Geometry check sheet. Reference: the model listing, model coordinates, mm. Face numbers are marked on the shaded views. A direction names the side the tool comes from. Give positions to 0.01 mm unless a question says otherwise; leave off trailing zeros. Order: outer loops, then holes, each group sorted by start corner. A loop starts at its lowest first (then second) coordinate and runs counter-clockwise, first axis right, second up.
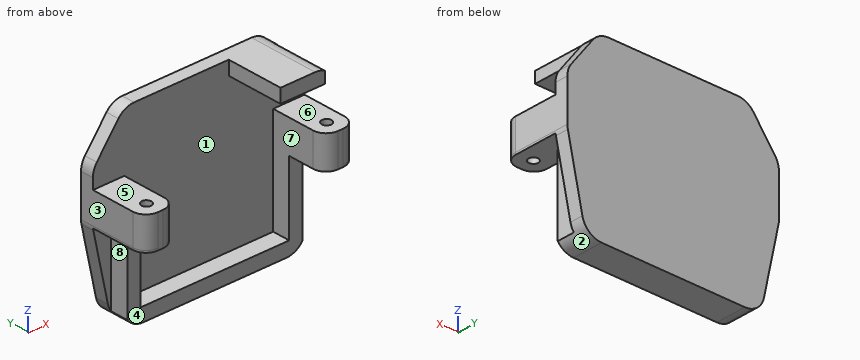
from build123d import *

# Parameters (mm, degrees)
BOSS_EXTRUDE1_START     = -14.7
BOSS_EXTRUDE1_OUTLINE_W = 32.4
BOSS_EXTRUDE1_OUTLINE_H = 27.1
BOSS_EXTRUDE1_DEPTH     = 14.7
CUT_EXTRUDE1_DEPTH      = 12.7
MOVE_FACE1_BY           = 4
MOVE_FACE1_2_BY         = 4
SKETCH3_W               = 2.8
SKETCH3_H               = 13.1
CUT_EXTRUDE2_DEPTH      = 13.7
CUT_EXTRUDE3_DEPTH      = 6
SKETCH5_R               = 0.75
CUT_EXTRUDE4_DEPTH      = 43.343439739
BOSS_EXTRUDE2_DEPTH     = 2
FILLET1_R               = 3
FILLET2_R               = 3
FILLET3_START           = -21
FILLET3_DEPTH           = 13
FILLET4_START           = -21
FILLET4_DEPTH           = 13
FILLET5_R               = 3
FILLET6_R               = 3
FILLET7_R               = 2


with BuildPart() as part:
    # Boss-Extrude1: read off the stored shape, not the designer's step
    # Boss-Extrude1 outline → Boss-Extrude1 (new body)
    with BuildSketch(Plane.XZ.offset(24.012143299).offset(BOSS_EXTRUDE1_START)):
        with Locations((16.432361385, -27.739579566)):
            Rectangle(BOSS_EXTRUDE1_OUTLINE_W, BOSS_EXTRUDE1_OUTLINE_H)
    extrude(amount=BOSS_EXTRUDE1_DEPTH)

    # Sketch2 → Cut-Extrude1 (cut)
    with BuildSketch(Plane.XZ.offset(24.012143299)):
        Polygon((27.832361385, -23.189579566), (32.632361385, -23.189579566), (32.632361385, -20.589579566), (27.832361385, -20.589579566), (27.832361385, -16.289579566), (5.032361385, -16.289579566), (5.032361385, -20.589579566), (0.232361385, -20.589579566), (0.232361385, -23.189579566), (5.032361385, -23.189579566), (5.032361385, -39.189579566), (27.832361385, -39.189579566), align=None)
    extrude(amount=-CUT_EXTRUDE1_DEPTH, mode=Mode.SUBTRACT)

    # Move Face1: a face moved inward by 4.0
    extrude(part.faces().sort_by_distance((16.432361385, -24.012143299, -39.479579566))[0], amount=MOVE_FACE1_BY, dir=(0, 1, 0), mode=Mode.SUBTRACT)

    # Move Face1 2: a face moved inward by 4.0
    extrude(part.faces().sort_by_distance((16.432361385, -24.012143299, -15.789579566))[0], amount=MOVE_FACE1_2_BY, dir=(0, 1, 0), mode=Mode.SUBTRACT)

    # Sketch3 → Cut-Extrude2 (cut)
    with BuildSketch(Plane.XZ.offset(20.012143299)):
        with Locations((1.632361385, -34.739579566)):
            Rectangle(SKETCH3_W, SKETCH3_H)
        with Locations((31.232361385, -34.739579566)):
            Rectangle(SKETCH3_W, SKETCH3_H)
        Polygon((0.232361385, -20.589579566), (5.032361385, -20.589579566), (5.032361385, -16.289579566), (21.032361385, -16.289579566), (21.032361385, -14.189579566), (0.232361385, -14.189579566), align=None)
        Polygon((27.832361385, -14.189579566), (32.632361385, -14.189579566), (32.632361385, -20.589579566), (27.832361385, -20.589579566), (27.832361385, -16.289579566), align=None)
    extrude(amount=-CUT_EXTRUDE2_DEPTH, mode=Mode.SUBTRACT)

    # Sketch4 → Cut-Extrude3 (cut)
    with BuildSketch(Plane.XZ.offset(20.012143299)):
        Polygon((3.032361385, -28.189579566), (5.032361385, -28.189579566), (5.032361385, -39.189579566), (27.832361385, -39.189579566), (27.832361385, -28.189579566), (29.832361385, -28.189579566), (29.832361385, -41.289579566), (3.032361385, -41.289579566), align=None)
    extrude(amount=-CUT_EXTRUDE3_DEPTH, mode=Mode.SUBTRACT)

    # Sketch5 → Cut-Extrude4 (cut, through all)
    with BuildSketch(Plane.XY.offset(-23.189579566)):
        with Locations((2.632361385, -17.662143299)):
            Circle(SKETCH5_R)
        with Locations((30.232361385, -17.662143299)):
            Circle(SKETCH5_R)
    extrude(amount=-CUT_EXTRUDE4_DEPTH, mode=Mode.SUBTRACT)

    # Sketch6 → Boss-Extrude2 (add)
    with BuildSketch(Plane(origin=(0, -9.312143299, 0), x_dir=(1, 0, 0), z_dir=(0, 1, 0))):
        Polygon((21.032361385, 14.189579566), (5.032361385, 14.189579566), (0.232361385, 20.589579566), (5.032361385, 20.589579566), (5.032361385, 16.289579566), (21.032361385, 16.289579566), align=None)
        Polygon((0.232361385, 28.189579566), (3.032361385, 41.289579566), (3.032361385, 28.189579566), align=None)
        Polygon((29.832361385, 41.289579566), (29.832361385, 28.189579566), (32.632361385, 28.189579566), align=None)
        Polygon((27.832361385, 20.589579566), (27.832361385, 14.189579566), (32.632361385, 20.589579566), align=None)
    extrude(amount=-BOSS_EXTRUDE2_DEPTH)

    # Fillet1
    # the kernel refuses this fillet: 3 mm, written as the material it takes off along each edge
    with BuildSketch(Plane(origin=(29.832361385, -17.378495337, -41.289579566), x_dir=(0.20901925718607187, 0, 0.9779115246919747), z_dir=(0, 1, 0))) as fillet1_piece_1:
        with BuildLine():
            CenterArc((FILLET1_R * 0.808846938434, -FILLET1_R), FILLET1_R, 90, 77.935115589)
            Line((-FILLET1_R * 0.169064586258, -FILLET1_R * 0.790980742814), (0, 0))
            Line((0, 0), (FILLET1_R * 0.808846938434, 0))
        make_face()
    extrude(amount=14.132704077, mode=Mode.SUBTRACT)

    # Fillet2
    # the kernel refuses this fillet: 3 mm, written as the material it takes off along each edge
    with BuildSketch(Plane(origin=(3.032361385, -17.378495337, -41.289579566), x_dir=(1.0, 0, -8.828560948914946e-12), z_dir=(0, 1, 0))) as fillet2_piece_1:
        with BuildLine():
            CenterArc((FILLET2_R * 0.808846938434, -FILLET2_R), FILLET2_R, 89.999999999, 77.935115589)
            Line((-FILLET2_R * 0.169064586256, -FILLET2_R * 0.790980742805), (0, 0))
            Line((0, 0), (FILLET2_R * 0.808846938443, 0))
        make_face()
    extrude(amount=14.132704077, mode=Mode.SUBTRACT)

    # Fillet3: read off the stored shape, not the designer's step
    # Fillet3 outline → Fillet3 (cut)
    with BuildSketch(Plane(origin=(0, 0, 0), x_dir=(1, 0, 0), z_dir=(0, 1, 0)).offset(FILLET3_START)):
        with BuildLine():
            Line((0.232361385, 28.189579566), (0.232361385, 27.872549323))
            ThreePointArc((0.232361385, 27.872549323), (0.248973736, 28.187824027), (0.29862681, 28.499607094))
            Line((0.29862681, 28.499607094), (0.232361385, 28.189579566))
        make_face()
    extrude(amount=FILLET3_DEPTH, mode=Mode.SUBTRACT)

    # Fillet4: read off the stored shape, not the designer's step
    # Fillet4 outline → Fillet4 (cut)
    with BuildSketch(Plane(origin=(0, 0, 0), x_dir=(1, 0, 0), z_dir=(0, 1, 0)).offset(FILLET4_START)):
        with BuildLine():
            Line((32.632361385, 28.189579566), (32.566095959, 28.499607094))
            ThreePointArc((32.566095959, 28.499607094), (32.615749033, 28.187824027), (32.632361385, 27.872549323))
            Line((32.632361385, 27.872549323), (32.632361385, 28.189579566))
        make_face()
    extrude(amount=FILLET4_DEPTH, mode=Mode.SUBTRACT)

    # Fillet5
    fillet5_edges = [part.edges().sort_by_distance(p)[0] for p in [
        (32.632361385, -10.312143299, -20.589579566),
        (5.032361385, -10.312143299, -14.189579566),
        (0.232361385, -10.312143299, -20.589579566),
    ]]
    fillet(fillet5_edges, radius=FILLET5_R)

    # Fillet6
    # the kernel refuses this fillet: 3 mm, written as the material it takes off along each edge
    with BuildSketch(Plane(origin=(27.832361385, -20.312143299, -14.189579566), x_dir=(-1.0, 0, -1.4283093226823923e-11), z_dir=(0, 1, 0))) as fillet6_piece_1:
        with BuildLine():
            CenterArc((FILLET6_R * 0.500000000009, -FILLET6_R), FILLET6_R, 90.000000001, 53.130102354)
            Line((-FILLET6_R * 0.3, -FILLET6_R * 0.400000000011), (-FILLET6_R * 0.316, -FILLET6_R * 0.388000000012))
            Line((-FILLET6_R * 0.316, -FILLET6_R * 0.388000000012), (-FILLET6_R * 0.0100000000003, FILLET6_R * 0.0199999999999))
            Line((-FILLET6_R * 0.0100000000003, FILLET6_R * 0.0199999999999), (FILLET6_R * 0.499999999994, FILLET6_R * 0.02))
            Line((FILLET6_R * 0.499999999994, FILLET6_R * 0.02), (FILLET6_R * 0.499999999995, 0))
        make_face()
    extrude(amount=20, mode=Mode.SUBTRACT)

    # Fillet7
    fillet7_edges = [part.edges().sort_by_distance(p)[0] for p in [
        (0.232361385, -20.012143299, -25.531064444),
        (27.832361385, -20.012143299, -25.689579566),
        (0.236563927, -20.012143299, -28.031286811),
        (32.632361385, -20.012143299, -25.531064444),
        (32.628158843, -20.012143299, -28.031286811),
        (5.032361385, -20.012143299, -25.689579566),
    ]]
    fillet(fillet7_edges, radius=FILLET7_R)


solid = part.part
Item 1: Sectioned sample at B-B (z = -27). Enter the section's corners in (x, y).
Reported:
outline: (0.23, -18.01) arc R2 ccw to (2.23, -20.01) - (3.03, -20.01) arc R2 ccw to (5.03, -18.01) - (5.03, -11.31) - (27.83, -11.31) - (27.83, -18.01) arc R2 ccw to (29.83, -20.01) - (30.63, -20.01) arc R2 ccw to (32.63, -18.01) - (32.63, -9.31) - (0.23, -9.31) - close; hole circle Ø1.5 at (2.63, -17.66); hole circle Ø1.5 at (30.23, -17.66)
Item 2: Sectioned sample at C-C (x = 25.5). Enter the section's corners in (y, z), and give its area (3 significant figures).
Reported:
outline: (-20.01, -16.29) - (-11.31, -16.29) - (-11.31, -39.19) - (-14.01, -39.19) - (-14.01, -41.29) - (-9.31, -41.29) - (-9.31, -14.19) - (-20.01, -14.19) - close
area: 78.1 mm2
Item 3: Set-up check for the marked faces 1, 2, 3, 4 and 5: record each of +Z, -Z, +X, -X, +Y, -Y from which the full face is reachable in a straight line by a thin tool's end or side.
Reported:
face 1: -Y
face 2: -Z, +X, +Y, -Y
face 3: +Z, -Z, -X, +Y, -Y
face 4: -Z, +X, -X, -Y
face 5: +Z, +X, -X, -Y
Item 4: Scan lines: L1, parallel to X at y = -11.75, z = -26; L2, parallel to Z at x = 25.5, y = -11.75; L3, parallel to X at y = -12.5, z = -34.75. Record each from-to range of solid material in increasing order.
Reported:
L1: x = 0.23 to 5.03, 27.83 to 32.63
L2: z = -41.29 to -39.19, -16.29 to -14.19
L3: x = 3.03 to 5.03, 27.83 to 29.83
Item 5: Sectioned sample at D-D (y = -10.5). Enter the section's corners in (x, z), and give its area (3 significant figures).
Reported:
outline: (0.23, -27.87) arc R3 ccw to (0.3, -28.5) - (2.53, -38.92) arc R3 ccw to (5.46, -41.29) - (27.41, -41.29) arc R3 ccw to (30.34, -38.92) - (32.57, -28.5) arc R3 ccw to (32.63, -27.87) - (32.63, -21.59) arc R3 ccw to (32.03, -19.79) - (28.73, -15.39) arc R3 ccw to (26.33, -14.19) - (6.53, -14.19) arc R3 ccw to (4.13, -15.39) - (0.83, -19.79) arc R3 ccw to (0.23, -21.59) - close
area: 807 mm2
Item 6: Gauge pin test, flat ends, axial feed: pin 1 (5.5 mm diameter, centred on x = 31, y = -15.5, fed in from -Z); pin 2 (1.4 mm diameter, centred on x = 3.5, y = -15.5, fed in from +Z); pin 3 (6.5 mm diameter, centred on x = 10.5, z = -36.5, fed in from -Y); pin 4 (2 mm diameter, centred on y = -14, z = -20.5, fed in from +X). Record the tip position at first contact, or that the pin passes through.
Reported:
pin 1: stops at z = -41
pin 2: stops at z = -23.19
pin 3: stops at y = -14.01
pin 4: passes through
Item 7: Draft check along X on the marked faces 6, 7 and 8. Enter one of: released by +X, released by -X, zero draft, split by the parting line, or undercut.
Reported:
face 6: zero draft
face 7: undercut
face 8: released by -X
Item 8: Sectioned sample at A-A (y = -14.5). Enter the section's corners in (x, z), and give its area (3 significant figures).
Reported:
outline: (0.23, -27.87) arc R3 ccw to (0.25, -28.19) - (5.03, -28.19) - (5.03, -23.19) - (0.23, -23.19) - close; (21.03, -16.29) - (27.83, -16.29) - (27.83, -14.59) arc R3 ccw to (26.33, -14.19) - (21.03, -14.19) - close; (27.83, -28.19) - (32.62, -28.19) arc R3 ccw to (32.63, -27.87) - (32.63, -23.19) - (27.83, -23.19) - close
area: 62.1 mm2
